Geometry: see drawing. Coordinates: mm, zero at the bounding-box minimum. A direction names the side the tool comes from. Give positions to 0.01 mm unless a question says otherwise; leave off trailing zeros. Loops run counter-clockwise (first coordinate to the right, second up) from the corner with the lowest first, then second, coordinate; pieces in that order, holes last. Notation, with made-up numbers: (89.25, -32.75) - (134.25, -32.75) arc R16 cw to (134.25, -23.75) - close; hole circle Ø11 at (-31.75, -7.5). An arc over 180 degrees is marked (long way). Use CSV: the item, a comma, the result in double quotes. Start each with the question number.
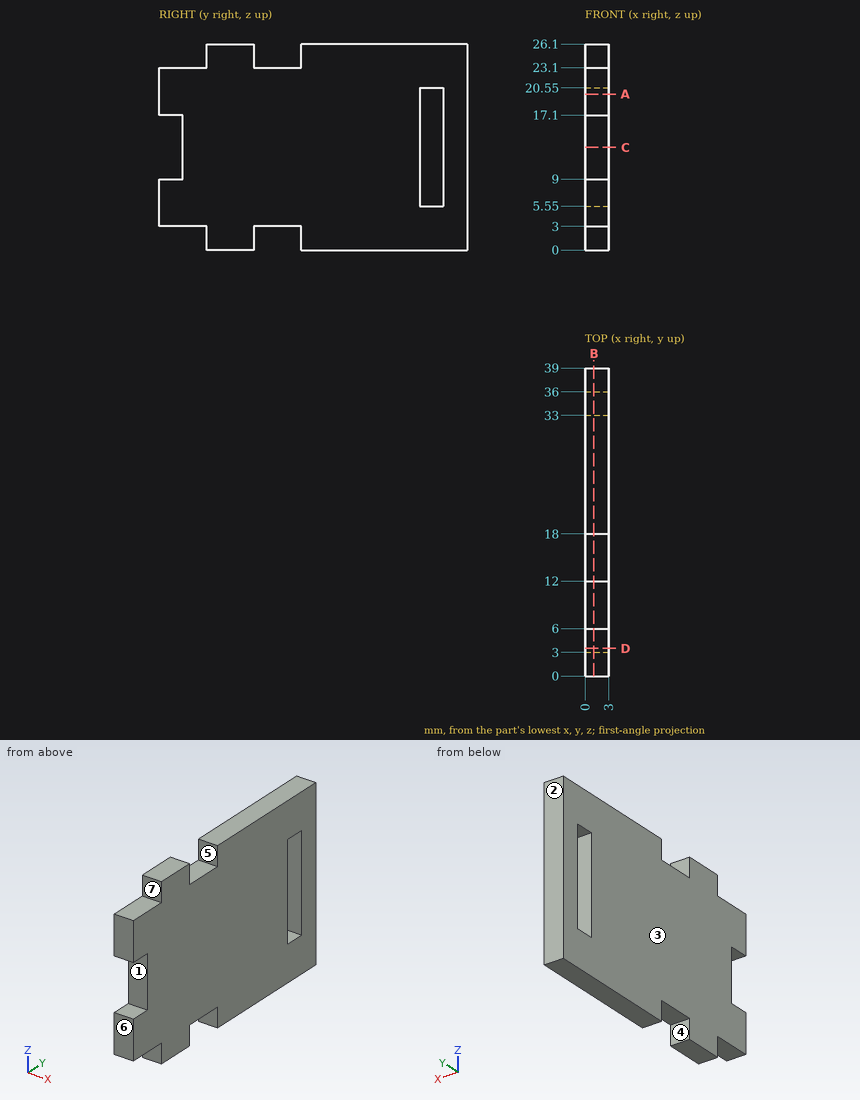
Item 1: Mould query, pull axis Z, two halves, no side actions, for the marked faces 1 and 2. Classes: pulls with the +Z half, pulls with the -Z half, needs draft (parallel to the pull), parting line crosses it, or undercut.
Item 2: Ray query, probe 1 along Y at (x, z) = (0.3, 1); probe 2 along Y at (x, z) = (0.7, 18); probe 3 along Z at (x, y) = (1.8, 17.5). Return the intervals inside material, ascending.
Item 3: Reachability of the marked faces 3, 4, 5, 6 and 7 from +Z, -Z, +X, -X, +Y, -Y: full face, straight path, thin tool, end or side. Return the list, or none.
Item 4: Pin query (flat end, axial travel): pin 1 Ø1.5 at (x, z) = (2, 1.5) entering from -Y; pin 2 Ø1.5 at (x, y) = (1.5, 1) entering from +Z; pin 3 Ø1.5 at (x, y) = (1, 14.5) entering from -Z. Return the tip coordinate at first contact, or that it passes through.
Item 5: Section C-C (z = 13). Output: boundary loops of the cut face in (x, y), plus the area to 3 significant figures.
Item 6: Section D-D (y = 3.5). Output: boundary loops of the cut face in (x, z), plus the area to 3 significant figures.
Item 7: Section B-B (x = 1.1). Output: boundary loops of the cut face in (y, z), plus the area to 3 significant figures.
Item 8: Section A-A (z = 19.75). Output: boundary loops of the cut face in (x, y), plus the area to 3 significant figures.
Outcome:
1,face 1,"undercut"
1,face 2,"needs draft"
2,probe 1,"y = 6 to 12, 18 to 39"
2,probe 2,"y = 0 to 33, 36 to 39"
2,probe 3,"z = 3 to 23.1"
3,face 3,"+Z, -Z, -X, +Y, -Y"
3,face 4,"-Z, +X, -X"
3,face 5,"+Z, +X, -X"
3,face 6,"+Z, -Z, +X, -X, -Y"
3,face 7,"+Z, +X, -X, -Y"
4,pin 1,"stops at y = 6"
4,pin 2,"stops at z = 23.1"
4,pin 3,"stops at z = 3"
5,outline,"(0, 3) - (3, 3) - (3, 33) - (0, 33) - close; (0, 36) - (3, 36) - (3, 39) - (0, 39) - close"
5,area,"99.0 mm2"
6,outline,"(0, 3) - (3, 3) - (3, 23.1) - (0, 23.1) - close"
6,area,"60.3 mm2"
7,outline,"(0, 3) - (6, 3) - (6, 0) - (12, 0) - (12, 3) - (18, 3) - (18, 0) - (39, 0) - (39, 26.1) - (18, 26.1) - (18, 23.1) - (12, 23.1) - (12, 26.1) - (6, 26.1) - (6, 23.1) - (0, 23.1) - (0, 17.1) - (3, 17.1) - (3, 9) - (0, 9) - close; hole (33, 5.55) - (36, 5.55) - (36, 20.55) - (33, 20.55) - close"
7,area,"877 mm2"
8,outline,"(0, 0) - (3, 0) - (3, 33) - (0, 33) - close; (0, 36) - (3, 36) - (3, 39) - (0, 39) - close"
8,area,"108 mm2"
